Read the model definition and answer for the solid it produces. Units are mm, in the model's axes. A direction names the side the tool comes from. Coordinates: 2 decimals unless noted, no trailing zeros. Loops run counter-clockwise (first coordinate to the right, second up) from the corner with the lowest first, then second, coordinate; pieces in that order, holes last. Notation, with made-up numbers: (89, -22.5) -> (129, -22.5) arc R30 cw to (129, 2.5) -> close; hole circle Ø8 at (68, 85). An arc over 180 degrees is marked (long way). Answer as a JSON object with one key per item and string values. Group by question number.
Q1. Determine the mould class of faces 1 (the flat face through (-1, 2, -1)), 2 (the cylindrical face through (-3.06, 0.99, 6.74)), 3 (the cylindrical face through (-22.999, 36.533, 41.486)), 4 (the cylindrical face through (-41.64, 0.9, -0.55)) for opening direction Y: released by +Y, released by -Y, zero draft, split by the parting line, or undercut.
Q2. Straight lines are drawn through the part: line 1 along Z through (x, y) = (-35, 9.5); line 2 along Y through (x, z) = (30, -3). For each, find the intervals that lie inside material, in ascending order. Write a range as [from, to].
Q3. The part is cut by section B-B on z = 0. Write down the section's boundary in (x, y), and give its area (3 significant figures).
Q4. The part is cut by section C-C on x = 0. Write down the section's boundary in (y, z).
Q5. The part is cut by section A-A on y = 4.5. Write down the section's boundary in (x, z).
Q6. For faces 5 (the flat face through (40.5, 16, -8)), 6 (the cylindrical face through (41.51, 40.9, -33.86)), 7 (the cylindrical face through (41.64, 26.83, -41.6)), 8 (the cylindrical face through (-41.51, 35.96, 23.99)), determine the directions among +Z, -Z, +X, -X, +Y, -Y from which every point of the face is accessible in a straight line to the end or side of a thin tool.
Q7. The part is cut by section D-D on z = 17. Write down the section's boundary in (x, y).
Q8. Each of these flat-tipped pins is pushed along its axis until it touches: P1, Ø10, axis at y = 19.5, z = 12, coming from the -X side; P2, Ø8, axis at x = 22.5, z = -32.5, coming from the +Y side. Where does it stop, or does it pass through?
from build123d import *

# Parameters (mm, degrees)
SKETCH1_W               = 85
SKETCH1_H               = 85
BOSS_EXTRUDE1_DEPTH     = 50
FILLET1_R               = 3
SHELL2_T                = -2
SKETCH2_R               = 8
CUT_EXTRUDE1_DEPTH      = 50
CUT_EXTRUDE2_DEPTH      = 108.383657975
CUT_EXTRUDE2_DEPTH_BACK = 108.383657975
SKETCH3_R               = 13
SKETCH4_R               = 13
SKETCH4_R_2             = 3
CUT_EXTRUDE3_DEPTH      = 50
SKETCH5_R               = 13
CUT_EXTRUDE4_DEPTH      = 50


with BuildPart() as part:
    # Sketch1 → Boss-Extrude1 (new body)
    with BuildSketch(Plane(origin=(0, 0, 0), x_dir=(1, 0, 0), z_dir=(0, 1, 0))):
        Rectangle(SKETCH1_W, SKETCH1_H)
    extrude(amount=BOSS_EXTRUDE1_DEPTH)

    # Fillet1
    fillet1_edges = [part.edges().sort_by_distance(p)[0] for p in [
        (0, 0, 42.5),
        (-42.5, 0, 0),
        (0, 0, -42.5),
        (42.5, 0, 0),
        (42.5, 25, 42.5),
        (-42.5, 25, 42.5),
        (-42.5, 25, -42.5),
        (42.5, 25, -42.5),
    ]]
    fillet(fillet1_edges, radius=FILLET1_R)

    # Shell2
    shell2_openings = [part.faces().sort_by_distance(p)[0] for p in [
        (0, 50, 0),
    ]]
    offset(amount=SHELL2_T, openings=shell2_openings, kind=Kind.INTERSECTION)

    # Sketch2 → Cut-Extrude1 (cut)
    with BuildSketch(Plane.XZ):
        with Locations(Location((0, 14.13265191, 0), (0, 0, 270))):
            Circle(SKETCH2_R)
        with Locations(Location((0, -11.86734809, 0), (0, 0, 270))):
            Circle(SKETCH2_R)
    extrude(amount=-CUT_EXTRUDE1_DEPTH, mode=Mode.SUBTRACT)

    # Sketch3 → Cut-Extrude2 (cut, two sides: drawn at the far end of the back side and taken through both)
    with BuildSketch(Plane.XY.offset(42.5).offset(-CUT_EXTRUDE2_DEPTH_BACK)):
        with Locations(Location((-17, 25, 0), (0, 0, 180))):
            Circle(SKETCH3_R)
        with Locations(Location((17, 25, 0), (0, 0, 180))):
            Circle(SKETCH3_R)
    extrude(amount=CUT_EXTRUDE2_DEPTH + CUT_EXTRUDE2_DEPTH_BACK, mode=Mode.SUBTRACT)

    # Sketch4 → Cut-Extrude3 (cut)
    with BuildSketch(Plane(origin=(42.5, 0, 0), x_dir=(0, 0, -1), z_dir=(1, 0, 0))):
        with Locations((0, 26.5)):
            Circle(SKETCH4_R)
        with Locations((30.997938674, 40)):
            Circle(SKETCH4_R_2)
    extrude(amount=-CUT_EXTRUDE3_DEPTH, mode=Mode.SUBTRACT)

    # Sketch5 → Cut-Extrude4 (cut)
    with BuildSketch(Plane.ZY.offset(42.5)):
        with Locations((-17, 25)):
            Circle(SKETCH5_R)
        with Locations((17, 25)):
            Circle(SKETCH5_R)
    extrude(amount=-CUT_EXTRUDE4_DEPTH, mode=Mode.SUBTRACT)


solid = part.part
Final values:
{
 "1": {"face 1": "released by +Y", "face 2": "zero draft", "face 3": "undercut", "face 4": "released by -Y"},
 "2": {"line 1": "z = [-42.5, -40.5], [40.5, 42.5]", "line 2": "y = [0, 2]"},
 "3": {"outline": "(-42.5, 3) arc R3 ccw to (-39.5, 0) -> (39.5, 0) arc R3 ccw to (42.5, 3) -> (42.5, 13.5) -> (40.5, 13.5) -> (40.5, 3) arc R1 cw to (39.5, 2) -> (-39.5, 2) arc R1 cw to (-40.5, 3) -> (-40.5, 50) -> (-42.5, 50) -> close; (40.5, 39.5) -> (42.5, 39.5) -> (42.5, 50) -> (40.5, 50) -> close", "area": "307 mm2"},
 "4": {"outline": "(0, -39.5) arc R3 ccw to (3, -42.5) -> (50, -42.5) -> (50, -40.5) -> (3, -40.5) arc R1 cw to (2, -39.5) -> (2, -19.87) -> (0, -19.87) -> close; (0, -3.87) -> (2, -3.87) -> (2, 6.13) -> (0, 6.13) -> close; (0, 22.13) -> (2, 22.13) -> (2, 39.5) arc R1 cw to (3, 40.5) -> (50, 40.5) -> (50, 42.5) -> (3, 42.5) arc R3 ccw to (0, 39.5) -> close"},
 "5": {"outline": "(-42.5, -39.5) arc R3 ccw to (-39.5, -42.5) -> (39.5, -42.5) arc R3 ccw to (42.5, -39.5) -> (42.5, 39.5) arc R3 ccw to (39.5, 42.5) -> (-39.5, 42.5) arc R3 ccw to (-42.5, 39.5) -> close; hole (-40.5, -39.5) arc R1 ccw to (-39.5, -40.5) -> (39.5, -40.5) arc R1 ccw to (40.5, -39.5) -> (40.5, 39.5) arc R1 ccw to (39.5, 40.5) -> (-39.5, 40.5) arc R1 ccw to (-40.5, 39.5) -> close"},
 "6": {"face 5": "+Y", "face 6": "+X", "face 7": "-Z, +X, +Y, -Y", "face 8": "-X"},
 "7": {"outline": "(-42.5, 3) arc R3 ccw to (-39.5, 0) -> (-7.47, 0) -> (-7.47, 2) -> (-39.5, 2) arc R1 cw to (-40.5, 3) -> (-40.5, 12) -> (-42.5, 12) -> close; (-42.5, 38) -> (-40.5, 38) -> (-40.5, 50) -> (-42.5, 50) -> close; (7.47, 0) -> (39.5, 0) arc R3 ccw to (42.5, 3) -> (42.5, 50) -> (40.5, 50) -> (40.5, 3) arc R1 cw to (39.5, 2) -> (7.47, 2) -> close"},
 "8": {"P1": "stops at x = 40.5", "P2": "stops at y = 2"}
}
